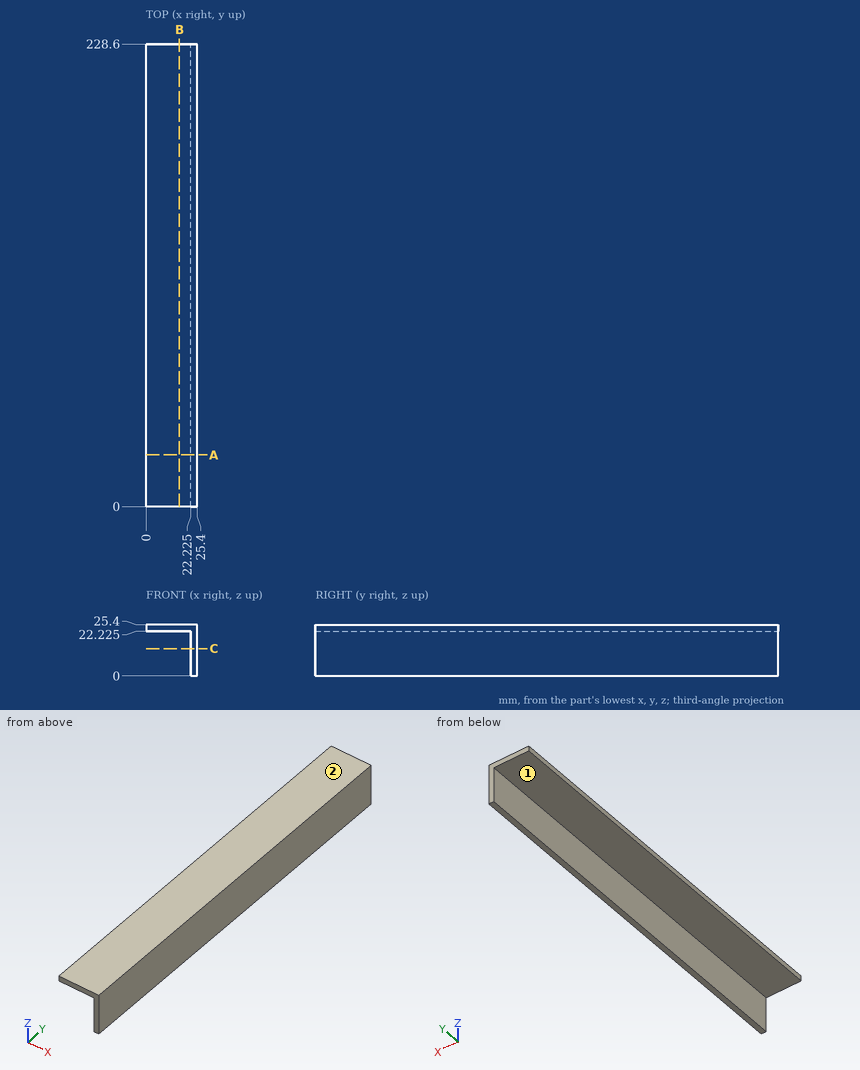
Part print with two shaded views. Sizes in mm from the minimum x, y, z corner. A direction names the side the tool comes from. Coordinates: 2 decimals unless noted, no trailing zeros. Write each loop counter-clockwise with the first axis right and the second up, starting at its lowest first coordinate (ties: lowest second). Pieces come first, ordered by that corner, then holes. Notation, with made-up numbers: (79, 61.25) - (110, 61.25) arc R34 cw to (110, 96.25) - close; hole circle Ø6 at (42.25, 25). An arc over 180 degrees is marked (long way). One line per item, written item: value. Start each with the question number.
1. Slice it at C-C (z = 13.5). Write the cut outline in (x, y) (3 decimals), plus the area to 3 significant figures.
2. Slice it at B-B (x = 16.5). Write the cut outline in (y, z) (3 decimals), plus the area to 3 significant figures.
3. Tool access for the marked faces 1 and 2: list every direction of +Z, -Z, +X, -X, +Y, -Y with a clear straight run to the whole face (end or side of a thin tool).
4. Probe line 1 (X direction, y = 56, z = 18.25) (3 decimals). List the from-to ranges inside material, lowest first. Write a range as from..to.
5. Flat gauge pins, fed straight in: pin 1 (11 mm diameter, centred on x = 8, y = 63, fed in from -Z) (3 decimals); pin 2 (6.5 mm diameter, centred on y = 112, z = 12, fed in from -X) (3 decimals). Where does each tip first touch, or does it go through?
6. Slice it at A-A (y = 25.5). Write the cut outline in (x, z) (3 decimals), plus the area to 3 significant figures.
Answers below:
1. outline: (22.225, 0) - (25.4, 0) - (25.4, 228.6) - (22.225, 228.6) - close
1. area: 726 mm^2
2. outline: (0, 22.225) - (228.6, 22.225) - (228.6, 25.4) - (0, 25.4) - close
2. area: 726 mm^2
3. face 1: -Z, -X, +Y, -Y
3. face 2: +Z, +X, -X, +Y, -Y
4. line 1: x = 22.225..25.4
5. pin 1: stops at z = 22.225
5. pin 2: stops at x = 22.225
6. outline: (0, 22.225) - (22.225, 22.225) - (22.225, 0) - (25.4, 0) - (25.4, 25.4) - (0, 25.4) - close
6. area: 151 mm^2
